```python
from build123d import *

# Parameters (mm, degrees)
SKETCH_1_R          = 67
SKETCH_1_R_2        = 17.55
EXTRUDE_1_DEPTH     = 2
EXTRUDE_START       = 18
SKETCH_2_R          = 67
SKETCH_2_R_2        = 31.2
EXTRUDE_2_DEPTH     = 18
FILLET_1_R          = 1
SHELL_4_T           = -2.5
SKETCH_4_R          = 0.85
EXTRUDE_3_DEPTH     = 18
FILLET_2_R          = 1
CUT_EXTRUDE_1_DEPTH = 1.2
SKETCH_6_R          = 64.5
CUT_EXTRUDE_2_DEPTH = 2


with BuildPart() as part:
    # 草图1 → 凸台-拉伸1 (new body)
    with BuildSketch(Plane.XY):
        Circle(SKETCH_1_R)
        Circle(SKETCH_1_R_2, mode=Mode.SUBTRACT)
    extrude(amount=EXTRUDE_1_DEPTH)

    # 草图2 → 凸台-拉伸2 (add)
    with BuildSketch(Plane(origin=(0, 0, 0), x_dir=(-1, 0, 0), z_dir=(0, 0, -1)).offset(EXTRUDE_START)):
        Circle(SKETCH_2_R)
        Circle(SKETCH_2_R_2, mode=Mode.SUBTRACT)
    extrude(amount=-EXTRUDE_2_DEPTH)

    # 圆角1
    fillet_1_edges = [part.edges().sort_by_distance(p)[0] for p in [
        (-67, 0, 2),
    ]]
    fillet(fillet_1_edges, radius=FILLET_1_R)

    # 抽壳4
    shell_4_openings = [part.faces().sort_by_distance(p)[0] for p in [
        (65.104953826, 0, -18),
    ]]
    offset(amount=SHELL_4_T, openings=shell_4_openings, kind=Kind.INTERSECTION)

    # 草图4 → 凸台-拉伸3 (add)
    # profile 1 of 6: a face of its own
    with BuildSketch(Plane(origin=(0, 0, 0), x_dir=(-1, 0, 0), z_dir=(0, 0, -1)).offset(EXTRUDE_START)):
        with BuildLine():
            Line((-41.05741952, 49.744731403), (-20.030225152, 27.101292964))
            ThreePointArc((-20.030225152, 27.101292964), (-23.785423834, 23.873491848), (-27.027081181, 20.130247958))
            Line((-27.027081181, 20.130247958), (-49.744731403, 41.05741952))
            ThreePointArc((-49.744731403, 41.05741952), (-45.608387387, 45.608387387), (-41.05741952, 49.744731403))
        make_face()
        with Locations(Location((-34, 34, 0), (0, 0, 180))):
            Circle(SKETCH_4_R, mode=Mode.SUBTRACT)
    # profile 2 of 6: a face of its own
    with BuildSketch(Plane(origin=(0, 0, 0), x_dir=(-1, 0, 0), z_dir=(0, 0, -1)).offset(EXTRUDE_START)):
        with BuildLine():
            Line((22.55149134, 60.42913402), (13.455295606, 30.897330308))
            ThreePointArc((13.455295606, 30.897330308), (8.782338501, 32.535527204), (3.919765525, 33.471262872))
            Line((3.919765525, 33.471262872), (10.684402617, 63.608910859))
            ThreePointArc((10.684402617, 63.608910859), (16.693828409, 62.302215796), (22.55149134, 60.42913402))
        make_face()
        with Locations(Location((12.444863729, 46.444863729, 0), (0, 0, 180))):
            Circle(SKETCH_4_R, mode=Mode.SUBTRACT)
    # profile 3 of 6: a face of its own
    with BuildSketch(Plane(origin=(0, 0, 0), x_dir=(-1, 0, 0), z_dir=(0, 0, -1)).offset(EXTRUDE_START)):
        with BuildLine():
            Line((63.608910859, 10.684402617), (33.485520759, 3.796037343))
            ThreePointArc((33.485520759, 3.796037343), (32.567762335, 8.662035356), (30.946846706, 13.341014914))
            Line((30.946846706, 13.341014914), (60.42913402, 22.55149134))
            ThreePointArc((60.42913402, 22.55149134), (62.302215796, 16.693828409), (63.608910859, 10.684402617))
        make_face()
        with Locations(Location((46.444863729, 12.444863729, 0), (0, 0, 180))):
            Circle(SKETCH_4_R, mode=Mode.SUBTRACT)
    # profile 4 of 6: a face of its own
    with BuildSketch(Plane(origin=(0, 0, 0), x_dir=(-1, 0, 0), z_dir=(0, 0, -1)).offset(EXTRUDE_START)):
        with BuildLine():
            Line((41.05741952, -49.744731403), (20.030225152, -27.101292964))
            ThreePointArc((20.030225152, -27.101292964), (23.785423834, -23.873491848), (27.027081181, -20.130247958))
            Line((27.027081181, -20.130247958), (49.744731403, -41.05741952))
            ThreePointArc((49.744731403, -41.05741952), (45.608387387, -45.608387387), (41.05741952, -49.744731403))
        make_face()
        with Locations(Location((34, -34, 0), (0, 0, 180))):
            Circle(SKETCH_4_R, mode=Mode.SUBTRACT)
    # profile 5 of 6: a face of its own
    with BuildSketch(Plane(origin=(0, 0, 0), x_dir=(-1, 0, 0), z_dir=(0, 0, -1)).offset(EXTRUDE_START)):
        with BuildLine():
            Line((-22.55149134, -60.42913402), (-13.455295606, -30.897330308))
            ThreePointArc((-13.455295606, -30.897330308), (-8.782338501, -32.535527204), (-3.919765525, -33.471262872))
            Line((-3.919765525, -33.471262872), (-10.684402617, -63.608910859))
            ThreePointArc((-10.684402617, -63.608910859), (-16.693828409, -62.302215796), (-22.55149134, -60.42913402))
        make_face()
        with Locations(Location((-12.444863729, -46.444863729, 0), (0, 0, 180))):
            Circle(SKETCH_4_R, mode=Mode.SUBTRACT)
    # profile 6 of 6: a face of its own
    with BuildSketch(Plane(origin=(0, 0, 0), x_dir=(-1, 0, 0), z_dir=(0, 0, -1)).offset(EXTRUDE_START)):
        with BuildLine():
            Line((-63.608910859, -10.684402617), (-33.485520759, -3.796037343))
            ThreePointArc((-33.485520759, -3.796037343), (-32.567762335, -8.662035356), (-30.946846706, -13.341014914))
            Line((-30.946846706, -13.341014914), (-60.42913402, -22.55149134))
            ThreePointArc((-60.42913402, -22.55149134), (-62.302215796, -16.693828409), (-63.608910859, -10.684402617))
        make_face()
        with Locations(Location((-46.444863729, -12.444863729, 0), (0, 0, 180))):
            Circle(SKETCH_4_R, mode=Mode.SUBTRACT)
    extrude(amount=-EXTRUDE_3_DEPTH)

    # 圆角2
    fillet_2_edges = [part.edges().sort_by_distance(p)[0] for p in [
        (67, 0, -18),
    ]]
    fillet(fillet_2_edges, radius=FILLET_2_R)

    # 草图5 → 切除-拉伸1 (cut)
    with BuildSketch(Plane(origin=(0, 0, -0.5), x_dir=(-1, 0, 0), z_dir=(0, 0, -1))):
        with BuildLine():
            Line((-63.608910859, -10.684402617), (-33.485520759, -3.796037343))
            ThreePointArc((-33.485520759, -3.796037343), (-32.535527204, 8.782338501), (-27.027081181, 20.130247958))
            Line((-27.027081181, 20.130247958), (-49.744731403, 41.05741952))
            ThreePointArc((-49.744731403, 41.05741952), (-62.302215796, 16.693828409), (-63.608910859, -10.684402617))
        make_face()
        with BuildLine():
            Line((-41.05741952, 49.744731403), (-20.030225152, 27.101292964))
            ThreePointArc((-20.030225152, 27.101292964), (-8.662035356, 32.567762335), (3.919765525, 33.471262872))
            Line((3.919765525, 33.471262872), (10.684402617, 63.608910859))
            ThreePointArc((10.684402617, 63.608910859), (-16.693828409, 62.302215796), (-41.05741952, 49.744731403))
        make_face()
        with BuildLine():
            Line((30.946846706, 13.341014914), (60.42913402, 22.55149134))
            ThreePointArc((60.42913402, 22.55149134), (45.608387387, 45.608387387), (22.55149134, 60.42913402))
            Line((22.55149134, 60.42913402), (13.455295606, 30.897330308))
            ThreePointArc((13.455295606, 30.897330308), (23.873491848, 23.785423834), (30.946846706, 13.341014914))
        make_face()
        with BuildLine():
            Line((27.027081181, -20.130247958), (49.744731403, -41.05741952))
            ThreePointArc((49.744731403, -41.05741952), (62.302215796, -16.693828409), (63.608910859, 10.684402617))
            Line((63.608910859, 10.684402617), (33.485520759, 3.796037343))
            ThreePointArc((33.485520759, 3.796037343), (32.535527204, -8.782338501), (27.027081181, -20.130247958))
        make_face()
        with BuildLine():
            Line((-3.919765525, -33.471262872), (-10.684402617, -63.608910859))
            ThreePointArc((-10.684402617, -63.608910859), (16.693828409, -62.302215796), (41.05741952, -49.744731403))
            Line((41.05741952, -49.744731403), (20.030225152, -27.101292964))
            ThreePointArc((20.030225152, -27.101292964), (8.662035356, -32.567762335), (-3.919765525, -33.471262872))
        make_face()
        with BuildLine():
            Line((-30.946846706, -13.341014914), (-60.42913402, -22.55149134))
            ThreePointArc((-60.42913402, -22.55149134), (-45.608387387, -45.608387387), (-22.55149134, -60.42913402))
            Line((-22.55149134, -60.42913402), (-13.455295606, -30.897330308))
            ThreePointArc((-13.455295606, -30.897330308), (-23.873491848, -23.785423834), (-30.946846706, -13.341014914))
        make_face()
    extrude(amount=-CUT_EXTRUDE_1_DEPTH, mode=Mode.SUBTRACT)

    # 草图6 → 切除-拉伸2 (cut)
    with BuildSketch(Plane(origin=(0, 0, -18), x_dir=(-1, 0, 0), z_dir=(0, 0, -1))):
        Circle(SKETCH_6_R)
    extrude(amount=-CUT_EXTRUDE_2_DEPTH, mode=Mode.SUBTRACT)


solid = part.part
```
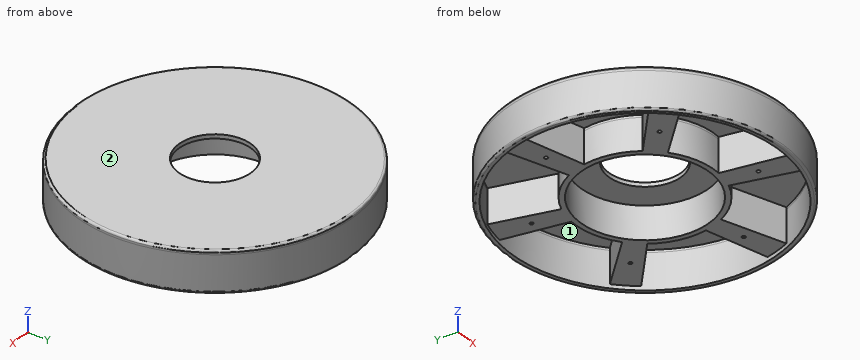
Source: CAD feature listing. Evaluate the final solid. Frame: model axes, mm. Face numbers are marked on the shaded views. Give positions to 0.01 mm unless a question says otherwise; leave off trailing zeros. Loops run counter-clockwise (first coordinate to the right, second up) from the corner with the lowest first, then second, coordinate; pieces in that order, holes last. Notation, with made-up numbers: (49.5, -9.5) -> (91.5, -9.5) arc R28 ccw to (91.5, 28.5) -> close; hole circle Ø11 at (31, 26). An arc over 180 degrees is marked (long way). Use a Markdown table: item, result. Add a question column.
(1) Pull-direction query (Y, two-part tool) for the marked faces 1 and 2; classes: +Y half, -Y half, draft (parallel to the pull), parting line (faces both ways), or undercut.
(2) Section query A-A (y = 0). Output: boundary loops of the cut face in (x, z).
(3) Ray query, line 1 (Y direction, x = 0, z = -5); line 2 (X direction, y = 26, z = -3.25); line 3 (X direction, y = -44, z = -0.25). Return the intervals inside material, ascending.
(4) First-contact query: pin 1 Ø10 at (x, z) = (-13.5, -7.5) entering from +Y; pin 2 Ø8 at (x, y) = (0, -43) entering from -Z; pin 3 Ø0.5 at (x, y) = (-34, -34.5) entering from -Z. Flat tips, straight axial feed; report the tip coordinate or a pass-through.
Checked values:
| question | item | result |
|---|---|---|
| 1 | face 1 | undercut |
| 1 | face 2 | draft |
| 2 | outline | (-67, -17) arc R1 ccw to (-66, -18) -> (-64.5, -18) -> (-64.5, 0.7) -> (-33.7, 0.7) -> (-33.7, -16) -> (-31.2, -16) -> (-31.2, 0) -> (-17.55, 0) -> (-17.55, 2) -> (-66, 2) arc R1 ccw to (-67, 1) -> close; (17.55, 0) -> (31.2, 0) -> (31.2, -16) -> (33.7, -16) -> (33.7, 0.7) -> (64.5, 0.7) -> (64.5, -18) -> (66, -18) arc R1 ccw to (67, -17) -> (67, 1) arc R1 ccw to (66, 2) -> (17.55, 2) -> close |
| 3 | line 1 | -67 to -64.5, -33.7 to -31.2, 31.2 to 33.7, 64.5 to 67 |
| 3 | line 2 | -61.75 to -59.03, -21.44 to -17.25, 17.25 to 33.4, 59.03 to 61.75 |
| 3 | line 3 | -50.53 to -35.72, 6.28 to 17.49, 47.16 to 50.53 |
| 4 | pin 1 | y = 66.46 |
| 4 | pin 2 | z = 0.7 |
| 4 | pin 3 | z = -0.5 |
